Source: CAD feature listing. Evaluate the final solid. Frame: model axes, mm. Face numbers are marked on the shaded views. A direction names the side the tool comes from. Round coordinates to 2 decimals unless told otherwise and drop trailing zeros. Loops run counter-clockwise (first coordinate to the right, second up) from the corner with the lowest first, then second, coordinate; pieces in that order, holes last.
Item 1: Section query C-C on z = -1.5. Return loops of the section in (x, y), then the cut area to 3 significant figures.
Item 2: Section query B-B on z = 8. Return loops of the section in (x, y), then the cut area to 3 significant figures.
Item 3: First-contact query: P1, Ø5, axis at y = 0, z = 14, coming from the +X side; P2, Ø2.5, axis at x = 1.5, z = 5, coming from the +Y side. Flat tips, straight axial feed; report the tip coordinate or a pass-through.
Item 4: Section query D-D on x = -2.75. Return loops of the section in (y, z).
Item 5: Ray query, L1, parallel to Z at x = 0, y = -4.25; L2, parallel to Z at x = -4.45, y = 0; L3, parallel to Y at x = -3, z = 9. Return the intervals inside material, ascending.
Item 6: Access query for the marked faces 1 and 2. Directions: +Z, -Z, +X, -X, +Y, -Y. A direction counts if a zero-diameter tool reaches every point of the face in a straight line with its end or side. Return the directions, or none.
Item 7: Section query A-A on x = 0. Return loops of the section in (y, z).
```python
from build123d import *

# Parameters (mm, degrees)
EXTRUDE_1_DEPTH     = 17
SKETCH_2_R          = 1.6
CUT_EXTRUDE_1_DEPTH = 21.346989949
SKETCH_3_R          = 1.6
CUT_EXTRUDE_2_DEPTH = 21.346989949


with BuildPart() as part:
    # ｽｹｯﾁ1 → 押し出し-薄板1 (new, symmetric)
    with BuildSketch(Plane.XY):
        Polygon((5, -5), (-5, -5), (-5, 5), (-4, 5), (-4, -4), (5, -4), align=None)
    extrude(amount=EXTRUDE_1_DEPTH, both=True)

    # ｽｹｯﾁ2 → ｶｯﾄ - 押し出し1 (cut, through all)
    with BuildSketch(Plane.ZY.offset(5)):
        with Locations(Location((-14, 0, 0), (0, 0, 270))):
            Circle(SKETCH_2_R)
        with Locations(Location((14, 0, 0), (0, 0, 270))):
            Circle(SKETCH_2_R)
    extrude(amount=-CUT_EXTRUDE_1_DEPTH, mode=Mode.SUBTRACT)

    # ｽｹｯﾁ3 → ｶｯﾄ - 押し出し2 (cut, through all)
    with BuildSketch(Plane.XZ.offset(5)):
        with Locations((0, -8)):
            Circle(SKETCH_3_R)
        with Locations((0, 8)):
            Circle(SKETCH_3_R)
    extrude(amount=-CUT_EXTRUDE_2_DEPTH, mode=Mode.SUBTRACT)


solid = part.part
```
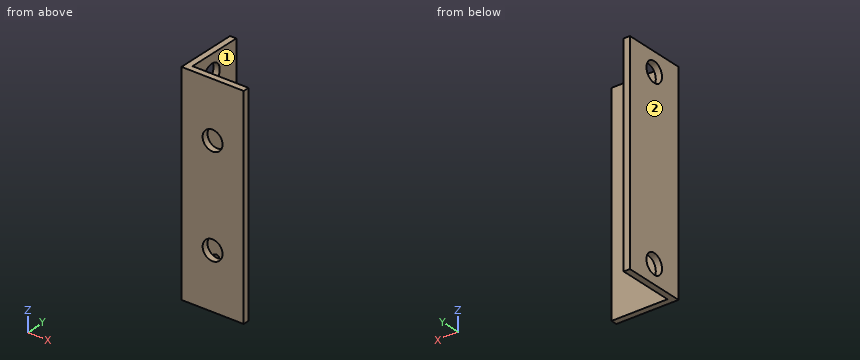
Data:
1. outline: (-5, -5) - (5, -5) - (5, -4) - (-4, -4) - (-4, 5) - (-5, 5) - close
1. area: 19.0 mm2
2. outline: (-5, -5) - (-1.6, -5) - (-1.6, -4) - (-4, -4) - (-4, 5) - (-5, 5) - close; (1.6, -5) - (5, -5) - (5, -4) - (1.6, -4) - close
2. area: 15.8 mm2
3. P1: stops at x = -4
3. P2: stops at y = -4
4. outline: (-5, -17) - (-4, -17) - (-4, 17) - (-5, 17) - close
5. L1: z = -17 to -9.6, -6.4 to 6.4, 9.6 to 17
5. L2: z = -17 to -15.6, -12.4 to 12.4, 15.6 to 17
5. L3: y = -5 to -4
6. face 1: +Z, -Z, +X, +Y
6. face 2: +Z, -Z, -X, +Y, -Y
7. outline: (-5, -17) - (-4, -17) - (-4, -9.6) - (-5, -9.6) - close; (-5, -6.4) - (-4, -6.4) - (-4, 6.4) - (-5, 6.4) - close; (-5, 9.6) - (-4, 9.6) - (-4, 17) - (-5, 17) - close
